Build history of the part. All positions in model axes, mm. A direction names the side the tool comes from. Round coordinates to 2 decimals unless told otherwise and drop trailing zeros. Loops run counter-clockwise (first coordinate to the right, second up) from the corner with the lowest first, then second, coordinate; pieces in that order, holes last. Notation, with made-up numbers: (36, 16) -> (93, 16) arc R25 ccw to (93, 43) -> close; hole circle Ø1 at (-23.75, 12). An arc over 180 degrees is marked (long way). Put each result on its own line as item: value. Start each with the question number.
Item 1: Cut at B-B, the plane x = 0. List the corners of the cut face in (y, z) (3 decimals).
Item 2: Drill centre lines: probe 1 along X at (y, z) = (-5, 101); probe 2 along Y at (x, z) = (-36, 66) (3 decimals); probe 3 along Z at (x, y) = (-14, -135) (3 decimals). Where is each one in solid material? Low to high. Write a range as [from, to].
Item 3: Flat gauge pins, fed straight in: pin 1 Ø2 at (x, z) = (15.5, 122.5) entering from -Y (3 decimals); pin 2 Ø2 at (x, y) = (-18.5, -60) entering from +Z (3 decimals). Where does each tip first touch, or does it go through?
Item 4: Cut at A-A, the plane y = -60.5. List the corners of the cut face in (x, z) (1 decimal).
Item 5: Cut at D-D, the plane x = 10. List the corners of the cut face in (y, z) (3 decimals).
Item 6: Pull direction X, two halves, no side cores. Call faces 4 (the flat face through (39.688, -43, 9)), 5 (the flat face through (-7.144, -80, 5)), 6 (the flat face through (9, -80, 9.525)): +X half, -X half, draft (parallel to the pull), parting line (faces both ways), or undercut.
Item 7: Tool access for faces 1 (the flat face through (1, -9.525, 82)), 2 (the flat face through (7.144, -80, 5)), 3 (the flat face through (1, 0, 75)): list every direction of +Z, -Z, +X, -X, +Y, -Y with a clear straight run to the whole face (end or side of a thin tool).
```python
from build123d import *

# Parameters (mm, degrees)
F1_DEPTH = 39.6875
F2_R     = 6.35
F3_DEPTH = 25.4
F4_W     = 14.2875
F4_H     = 77.7875
F5_DEPTH = 25.4


with BuildPart() as f1:
    # F0 (on Right) → F1 (new body, symmetric)
    with BuildSketch(Plane.YZ):
        with BuildLine():
            Line((0, 0), (0, 152.4))
            ThreePointArc((0, 152.4), (-6.7351920908, 149.6101920908), (-9.525, 142.875))
            Line((-9.525, 142.875), (-9.525, 19.05))
            ThreePointArc((-9.525, 19.05), (-12.3148079092, 12.3148079092), (-19.05, 9.525))
            Line((-19.05, 9.525), (-142.875, 9.525))
            ThreePointArc((-142.875, 9.525), (-149.6101920908, 6.7351920908), (-152.4, 0))
            Line((-152.4, 0), (0, 0))
        make_face()
    extrude(amount=F1_DEPTH, both=True)

    # F2 (on face) → F3 (cut)
    with BuildSketch(Plane(origin=(0, 0, 0), x_dir=(-1, 0, 0), z_dir=(0, 1, 0))):
        with Locations((0, 101.6)):
            Circle(F2_R)
    extrude(amount=-F3_DEPTH, mode=Mode.SUBTRACT)

    # F4 (on face) → F5 (cut)
    with BuildSketch(Plane(origin=(0, 0, 0), x_dir=(1, 0, 0), z_dir=(0, 0, -1))):
        with Locations((0, 80.9625)):
            Rectangle(F4_W, F4_H)
        with BuildLine():
            Line((-7.14375, 119.85625), (7.14375, 119.85625))
            ThreePointArc((7.14375, 119.85625), (0, 127), (-7.14375, 119.85625))
        make_face()
        with BuildLine():
            ThreePointArc((-7.14375, 42.06875), (0, 34.925), (7.14375, 42.06875))
            Line((7.14375, 42.06875), (-7.14375, 42.06875))
        make_face()
    extrude(amount=-F5_DEPTH, mode=Mode.SUBTRACT)


solid = f1.part
```
Reply:
1. outline: (-152.4, 0) -> (-127, 0) -> (-127, 9.525) -> (-142.875, 9.525) arc R9.525 ccw to start; (-34.925, 0) -> (0, 0) -> (0, 95.25) -> (-9.525, 95.25) -> (-9.525, 19.05) arc R9.525 cw to (-19.05, 9.525) -> (-34.925, 9.525) -> close; (-9.525, 107.95) -> (0, 107.95) -> (0, 152.4) arc R9.525 ccw to (-9.525, 142.875) -> close
2. probe 1: x = [-39.69, -6.32], [6.32, 39.69]
2. probe 2: y = [-9.525, 0]
2. probe 3: z = [0, 9.525]
3. pin 1: stops at y = -9.525
3. pin 2: stops at z = 9.525
4. outline: (-39.7, 0) -> (-7.1, 0) -> (-7.1, 9.5) -> (-39.7, 9.5) -> close; (7.1, 0) -> (39.7, 0) -> (39.7, 9.5) -> (7.1, 9.5) -> close
5. outline: (-152.4, 0) -> (0, 0) -> (0, 152.4) arc R9.525 ccw to (-9.525, 142.875) -> (-9.525, 19.05) arc R9.525 cw to (-19.05, 9.525) -> (-142.875, 9.525) arc R9.525 ccw to start
6. face 4: +X half
6. face 5: undercut
6. face 6: draft
7. face 1: +Z, +X, -X, -Y
7. face 2: +Z, -Z
7. face 3: +Z, -Z, +X, -X, +Y
